Study the drawing (mm; zero at the part's minimum x, y, z) and answer. A direction names the side the tool comes from. Coordinates: 2 decimals unless noted, no trailing zeros. Loops run counter-clockwise (first coordinate to the right, second up) from the corner with the lowest first, then second, coordinate; pieces in that order, holes last. Notation, with made-up numbers: (72.5, 66) - (129.5, 66) arc R18 cw to (129.5, 77) - close; hole circle Ø6 at (-2.5, 0). An arc over 180 degrees is marked (long way). Use one line per item in the form item = value.
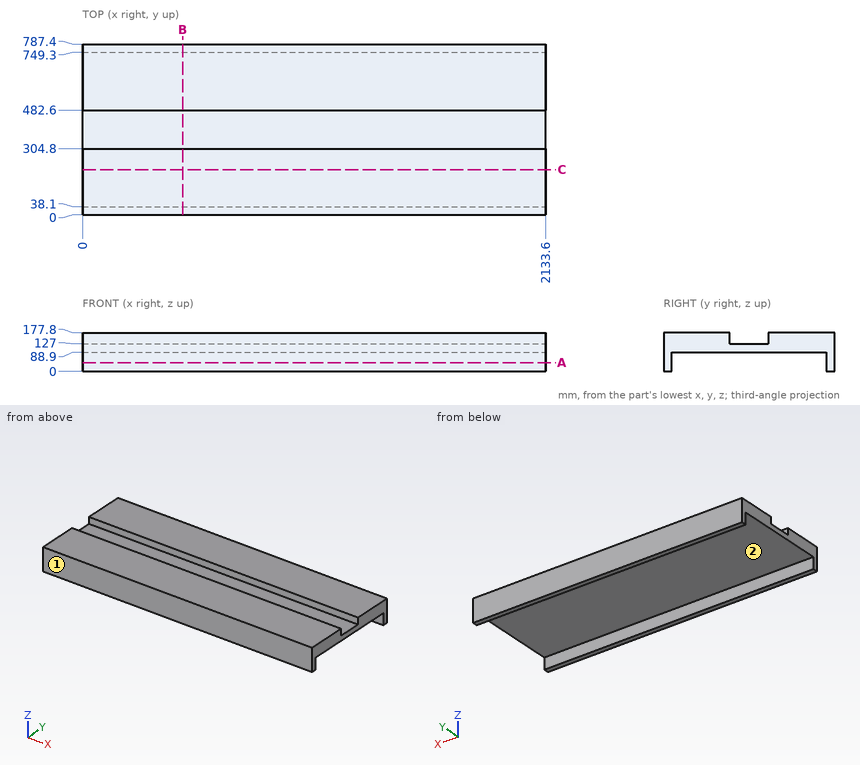
Item 1: The part is cut by section A-A on z = 41. Give the vertices of the cut face in (x, y), plus the area to 3 significant figures.
Results below:
outline = (0, 0) - (2133.6, 0) - (2133.6, 38.1) - (0, 38.1) - close; (0, 749.3) - (2133.6, 749.3) - (2133.6, 787.4) - (0, 787.4) - close
area = 163,000 mm²
Item 2: The part is cut by section C-C on y = 208.5. Give the vertices of the cut face in (x, z), plus the area to 3 significant figures.
Results below:
outline = (0, 88.9) - (2133.6, 88.9) - (2133.6, 177.8) - (0, 177.8) - close
area = 190,000 mm²
Item 3: Which of the six approach directions +Z, -Z, +X, -X, +Y, -Y give full straight-line access (tool end or side, diameter ignored) to the marked faces 1 and 2?
Results below:
face_1 = +Z, -Z, +X, -X, -Y
face_2 = -Z, +X, -X
Item 4: The part is cut by section B-B on x = 461. Give the vertices of the cut face in (y, z), plus the area to 3 significant figures.
Results below:
outline = (0, 0) - (38.1, 0) - (38.1, 88.9) - (749.3, 88.9) - (749.3, 0) - (787.4, 0) - (787.4, 177.8) - (482.6, 177.8) - (482.6, 127) - (304.8, 127) - (304.8, 177.8) - (0, 177.8) - close
area = 67,700 mm²
Item 5: Find the intervals of material crossed by L1, parallel to Y at x = 670, z = 77.5; L2, parallel to Y at x = 1247, z = 146; L3, parallel to Z at x = 1601.5, y = 655, in increasing order.
Results below:
L1 = 0 to 38.1, 749.3 to 787.4
L2 = 0 to 304.8, 482.6 to 787.4
L3 = 88.9 to 177.8
Item 6: Each of these flat-tipped pins is pushed along its axis until it touches: P1, Ø10, axis at x = 1029, y = 352, coming from the -Z side; P2, Ø3, axis at x = 764, y = 358.5, coming from the +Z side; P3, Ø3, axis at x = 1167, z = 87, coming from the -Y side. Where does it stop, or does it pass through?
Results below:
P1 = 88.9
P2 = 127
P3 = 0
